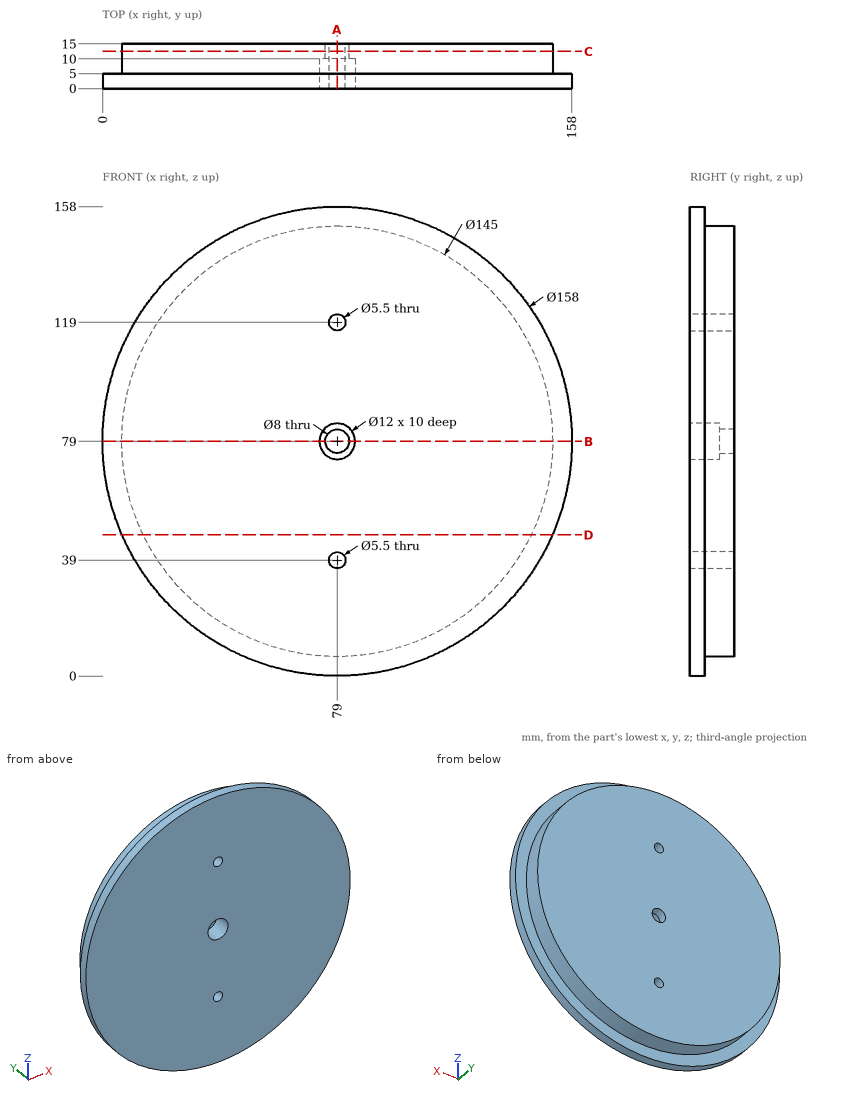
Check sheet for the drawn part. Datum: minimum x, y, z corner. Units: mm. Give positions to 0.01 mm unless a question says otherwise; leave off trailing zeros. Loops run counter-clockwise (first coordinate to the right, second up) from the corner with the lowest first, then second, coordinate; pieces in that order, holes last.
1) Sectioned sample at C-C, the plane y = 12.5. Enter the section's corners in (x, z), then the cut area to 3 significant figures.
2) Sectioned sample at D-D, the plane z = 47.5. Enter the section's corners in (x, y).
3) Sectioned sample at B-B, the plane z = 79. Enter the section's corners in (x, y), then the cut area to 3 significant figures.
4) Thickness scan on line 1 along X through (y, z) = (4.5, 79); line 2 along Y through (x, z) = (151, 63); line 3 along X through (y, z) = (3.5, 39). Record the ranges inside material, lowest first.
5) Depth check by flat-ended pin: pin 1 Ø1.5 at (x, y) = (107, 13.5) entering from -Z; pin 2 Ø6 at (x, y) = (42, 9.5) entering from +Z; pin 3 Ø1 at (y, z) = (7, 22) entering from -X. Enter the tip coordinate at first touch or a pass-through.
6) Sectioned sample at A-A, the plane x = 79. Enter the section's corners in (y, z).
Answers:
1. outline: circle Ø145 at (79, 79); hole circle Ø8 at (79, 79); hole circle Ø5.5 at (79, 39); hole circle Ø5.5 at (79, 119)
1. area: 16,400 mm2
2. outline: (6.55, 0) - (151.45, 0) - (151.45, 5) - (144.3, 5) - (144.3, 15) - (13.7, 15) - (13.7, 5) - (6.55, 5) - close
3. outline: (0, 0) - (73, 0) - (73, 10) - (75, 10) - (75, 15) - (6.5, 15) - (6.5, 5) - (0, 5) - close; (83, 10) - (85, 10) - (85, 0) - (158, 0) - (158, 5) - (151.5, 5) - (151.5, 15) - (83, 15) - close
3. area: 2,080 mm2
4. line 1: x = 0 to 73, 85 to 158
4. line 2: y = 0 to 5
4. line 3: x = 10.88 to 76.25, 81.75 to 147.12
5. pin 1: stops at z = 11.82
5. pin 2: stops at z = 143.03
5. pin 3: stops at x = 33.57
6. outline: (0, 0) - (5, 0) - (5, 6.5) - (15, 6.5) - (15, 36.25) - (0, 36.25) - close; (0, 41.75) - (15, 41.75) - (15, 75) - (10, 75) - (10, 73) - (0, 73) - close; (0, 85) - (10, 85) - (10, 83) - (15, 83) - (15, 116.25) - (0, 116.25) - close; (0, 121.75) - (15, 121.75) - (15, 151.5) - (5, 151.5) - (5, 158) - (0, 158) - close
